from build123d import *

# Parameters (mm, degrees)
SKETCH1_R           = 11
SKETCH1_R_2         = 1.95
BOSS_EXTRUDE1_DEPTH = 4
SKETCH2_R           = 5.1
BOSS_EXTRUDE2_DEPTH = 18.5
SKETCH3_R           = 6.925
BOSS_EXTRUDE3_DEPTH = 4
SKETCH4_R           = 4
CUT_EXTRUDE1_DEPTH  = 31.728651126


with BuildPart() as part:
    # Sketch1 → Boss-Extrude1 (new body)
    with BuildSketch(Plane(origin=(0, 0, 0), x_dir=(1, 0, 0), z_dir=(0, 1, 0))):
        with Locations(Location((0, 0, 0), (0, 0, 270))):
            Circle(SKETCH1_R)
        with Locations(Location((-8.2, 0, 0), (0, 0, 270))):
            Circle(SKETCH1_R_2, mode=Mode.SUBTRACT)
        with Locations(Location((8.2, 0, 0), (0, 0, 90))):
            Circle(SKETCH1_R_2, mode=Mode.SUBTRACT)
        with Locations(Location((0, 8.2, 0), (0, 0, 270))):
            Circle(SKETCH1_R_2, mode=Mode.SUBTRACT)
        with Locations(Location((0, -8.2, 0), (0, 0, 90))):
            Circle(SKETCH1_R_2, mode=Mode.SUBTRACT)
    extrude(amount=BOSS_EXTRUDE1_DEPTH)

    # Sketch2 → Boss-Extrude2 (add)
    with BuildSketch(Plane(origin=(0, 4, 0), x_dir=(1, 0, 0), z_dir=(0, 1, 0))):
        with Locations(Location((0, 0, 0), (0, 0, 270))):
            Circle(SKETCH2_R)
    extrude(amount=BOSS_EXTRUDE2_DEPTH)

    # Sketch3 → Boss-Extrude3 (add)
    with BuildSketch(Plane(origin=(0, 22.5, 0), x_dir=(1, 0, 0), z_dir=(0, 1, 0))):
        with Locations(Location((0, 0, 0), (0, 0, 270))):
            Circle(SKETCH3_R)
    extrude(amount=BOSS_EXTRUDE3_DEPTH)

    # Sketch4 → Cut-Extrude1 (cut, through all)
    with BuildSketch(Plane(origin=(0, 26.5, 0), x_dir=(1, 0, 0), z_dir=(0, 1, 0))):
        with Locations(Location((0, 0, 0), (0, 0, 270))):
            Circle(SKETCH4_R)
    extrude(amount=-CUT_EXTRUDE1_DEPTH, mode=Mode.SUBTRACT)


solid = part.part
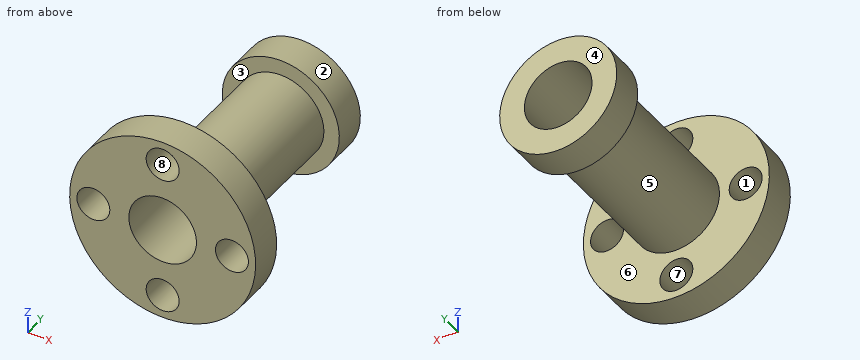
Work out the finished part from the listing and answer in its coordinate system (mm). Face numbers are marked on the shaded views. A direction names the side the tool comes from. Give positions to 0.01 mm unless a question says otherwise; leave off trailing zeros. Loops run counter-clockwise (first coordinate to the right, second up) from the corner with the lowest first, then second, coordinate; pieces in that order, holes last. Notation, with made-up numbers: (-12.75, -3.5) - (0.25, -3.5) arc R15 ccw to (0.25, 9.5) - close; hole circle Ø9 at (74.5, 53.5). An arc over 180 degrees is marked (long way). Answer in a Markdown table with one row per item. Add a question column.
Q1. The part is cut by section D-D (z = -8.2). Determine the outline of the cut face in (x, y), and give its area (3 significant figures).
Q2. Each of these flat-tipped pins is pushed along its axis until it touches: P1, Ø3.5, axis at x = -8.2, z = 0, coming from the -Y side; P2, Ø2, axis at y = 4, z = 1.5, coming from the -X side; P3, Ø1, axis at y = 11.5, z = -3, coming from the +X side. Where does it stop, or does it pass through?
Q3. Consider line 1 along X through (y, z) = (1.5, 0); line 2 along X through (y, z) = (16.75, 0); line 3 along Y through (x, z) = (3.25, 7.25). Determine where each line is inside the solid, lowest interval first.
Q4. The part is cut by section C-C (x = -9). Determine the outline of the cut face in (y, z), and give its area (3 significant figures).
Q5. The part is cut by section B-B (x = 0). Determine the outline of the cut face in (y, z) (3 decimals), and give its area (3 significant figures).
Q6. A tool of negligible diameter and unlimited length cuts with its end or side. For the marked faces 1, 2, 3 and 4, from which of +Z, -Z, +X, -X, +Y, -Y can it reach the whole face along a straight path? Write none if from no direction.
Q7. The part is cut by section A-A (z = 0). Determine the outline of the cut face in (x, y) (3 decimals).
Q8. Determine the mould class of the marked faces 5, 6, 7 and 8 for opening direction Z: released by +Z, released by -Z, zero draft, split by the parting line, or undercut.
Solution:
| question | item | result |
|---|---|---|
| 1 | outline | (-7.33, 0) - (-1.95, 0) - (-1.95, 4) - (-7.33, 4) - close; (1.95, 0) - (7.33, 0) - (7.33, 4) - (1.95, 4) - close |
| 1 | area | 43.1 mm² |
| 2 | P1 | stops at y = 22.5 |
| 2 | P2 | stops at x = -10.99 |
| 2 | P3 | stops at x = 4.45 |
| 3 | line 1 | x = -11 to -10.15, -6.25 to -4, 4 to 6.25, 10.15 to 11 |
| 3 | line 2 | x = -5.1 to -4, 4 to 5.1 |
| 3 | line 3 | y = 0 to 4 |
| 4 | outline | (0, -6.32) - (4, -6.32) - (4, -1.78) - (0, -1.78) - close; (0, 1.78) - (4, 1.78) - (4, 6.32) - (0, 6.32) - close |
| 4 | area | 36.4 mm² |
| 5 | outline | (0, -11) - (4, -11) - (4, -10.15) - (0, -10.15) - close; (0, -6.25) - (4, -6.25) - (4, -5.1) - (22.5, -5.1) - (22.5, -6.925) - (26.5, -6.925) - (26.5, -4) - (0, -4) - close; (0, 4) - (26.5, 4) - (26.5, 6.925) - (22.5, 6.925) - (22.5, 5.1) - (4, 5.1) - (4, 6.25) - (0, 6.25) - close; (0, 10.15) - (4, 10.15) - (4, 11) - (0, 11) - close |
| 5 | area | 88.9 mm² |
| 6 | face 1 | -Y |
| 6 | face 2 | +Y |
| 6 | face 3 | none |
| 6 | face 4 | +Z, -Z, +X, -X, +Y |
| 7 | outline | (-11, 0) - (-10.15, 0) - (-10.15, 4) - (-11, 4) - close; (-6.925, 22.5) - (-5.1, 22.5) - (-5.1, 4) - (-6.25, 4) - (-6.25, 0) - (-4, 0) - (-4, 26.5) - (-6.925, 26.5) - close; (4, 0) - (6.25, 0) - (6.25, 4) - (5.1, 4) - (5.1, 22.5) - (6.925, 22.5) - (6.925, 26.5) - (4, 26.5) - close; (10.15, 0) - (11, 0) - (11, 4) - (10.15, 4) - close |
| 8 | face 5 | split by the parting line |
| 8 | face 6 | zero draft |
| 8 | face 7 | undercut |
| 8 | face 8 | undercut |
